```python
from build123d import *

# Parameters (mm, degrees)
SKETCH_2_R          = 1.05
EXTRUDE_1_DEPTH     = 6
EXTRUDE_3_DEPTH     = 10
SKETCH_5_R          = 1.75
CUT_EXTRUDE_1_DEPTH = 20.293781382
SKETCH_6_W          = 13
SKETCH_6_H          = 13
CUT_EXTRUDE_2_DEPTH = 1.5


with BuildPart() as part:
    # 草图2 → 凸台-拉伸1 (new body)
    with BuildSketch(Plane(origin=(0, 0, 0), x_dir=(1, 0, 0), z_dir=(0, 1, 0))):
        Polygon((-6.5, 3.25), (6.5, 3.25), (6.5, -6.75), (3.5, -9.75), (-6.5, -9.75), align=None)
        with Locations(Location((-3.25, 0, 0), (0, 0, 270))):
            Circle(SKETCH_2_R, mode=Mode.SUBTRACT)
        with Locations(Location((3.25, 0, 0), (0, 0, 270))):
            Circle(SKETCH_2_R, mode=Mode.SUBTRACT)
        with Locations(Location((-3.25, -6.5, 0), (0, 0, 270))):
            Circle(SKETCH_2_R, mode=Mode.SUBTRACT)
    extrude(amount=EXTRUDE_1_DEPTH)

    # 草图4 → 凸台-拉伸3 (add)
    with BuildSketch(Plane(origin=(6.5, 0, 11.5), x_dir=(0, 0, -1), z_dir=(1, 0, 0))):
        Polygon((9.75, 6), (9.75, 4.5), (10.95, 4.5), (10.95, 1.5), (9.75, 1.5), (9.75, 0), (6.75, 0), (6.75, 6), align=None)
    extrude(amount=EXTRUDE_3_DEPTH)

    # 草图5 → 切除-拉伸1 (cut, through all)
    with BuildSketch(Plane.XY.offset(4.75)):
        with Locations((10.5, 3)):
            Circle(SKETCH_5_R)
    extrude(amount=-CUT_EXTRUDE_1_DEPTH, mode=Mode.SUBTRACT)

    # 草图6 → 切除-拉伸2 (cut)
    with BuildSketch(Plane(origin=(0, 6, 0), x_dir=(1, 0, 0), z_dir=(0, 1, 0))):
        with Locations((0, -3.25)):
            Rectangle(SKETCH_6_W, SKETCH_6_H)
    extrude(amount=-CUT_EXTRUDE_2_DEPTH, mode=Mode.SUBTRACT)


solid = part.part
```
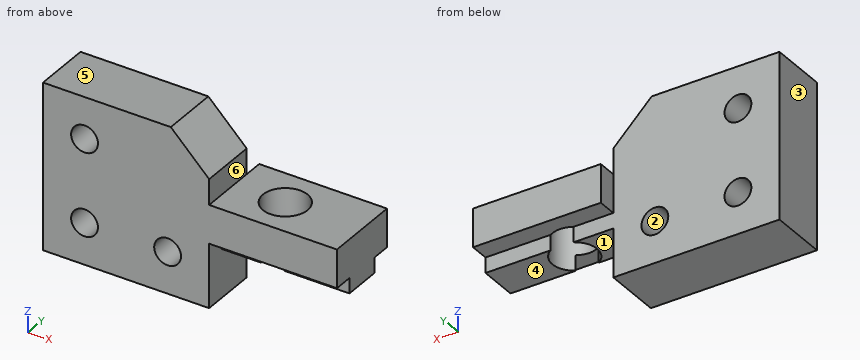
Geometry check sheet. Reference: the model listing, model coordinates, mm. Face numbers are marked on the shaded views. A direction names the side the tool comes from. Round coordinates to 2 decimals unless told otherwise and drop trailing zeros. Write each loop counter-clockwise with the first axis right and the second up, starting at its lowest first coordinate (ties: lowest second). Pieces come first, ordered by that corner, then holes. Notation, with made-up numbers: (6.25, -28) -> (32.25, -28) arc R18 ccw to (32.25, -7) -> close; hole circle Ø10 at (57, -18). An arc over 180 degrees is marked (long way). Put each result on its own line as item: value.
1) Cross-section at C-C, the plane z = 2.75. Enter the section's corners in (x, y).
Recorded:
outline: (-6.5, 0) -> (16.5, 0) -> (16.5, 6) -> (6.5, 6) -> (6.5, 4.5) -> (-6.5, 4.5) -> close; hole circle Ø3.5 at (10.5, 3)
2) Release check for a two-part mould opening along Z. For the marked faces 1, 2 and 3 record: pulls with the +Z half, pulls with the -Z half, needs draft (parallel to the pull), parting line crosses it, or undercut.
Recorded:
face 1: pulls with the -Z half
face 2: undercut
face 3: needs draft
3) Depth check by flat-ended pin: P1, Ø1, axis at y = 2.5, z = 6, coming from the +X side; P2, Ø4, axis at x = 3, z = 0, coming from the -Y side; P3, Ø1.3, axis at x = 14.5, z = 1, coming from the -Y side; P4, Ø2.5, axis at x = 14.5, y = 3, coming from the -Z side. Enter the tip coordinate at first touch or a pass-through.
Recorded:
P1: stops at x = 6.5
P2: stops at y = 0
P3: stops at y = 1.5
P4: stops at z = 0.55
4) Cross-section at A-A, the plane y = 3. Enter the section's corners in (x, z).
Recorded:
outline: (-6.5, -3.25) -> (6.5, -3.25) -> (6.5, 0.55) -> (8.75, 0.55) -> (8.75, 4.75) -> (6.5, 4.75) -> (6.5, 6.75) -> (3.5, 9.75) -> (-6.5, 9.75) -> close; (12.25, 0.55) -> (16.5, 0.55) -> (16.5, 4.75) -> (12.25, 4.75) -> close; hole circle Ø2.1 at (-3.25, 0); hole circle Ø2.1 at (-3.25, 6.5); hole circle Ø2.1 at (3.25, 0)
5) Cross-section at B-B, the plane x = 10.5. Enter the section's corners in (y, z).
Recorded:
outline: (0, 1.75) -> (1.25, 1.75) -> (1.25, 4.75) -> (0, 4.75) -> close; (4.75, 1.75) -> (6, 1.75) -> (6, 4.75) -> (4.75, 4.75) -> close
6) Cross-section at D-D, the plane y = 0.9. Enter the section's corners in (x, z).
Recorded:
outline: (-6.5, -3.25) -> (6.5, -3.25) -> (6.5, 1.75) -> (16.5, 1.75) -> (16.5, 4.75) -> (6.5, 4.75) -> (6.5, 6.75) -> (3.5, 9.75) -> (-6.5, 9.75) -> close; hole circle Ø2.1 at (-3.25, 0); hole circle Ø2.1 at (-3.25, 6.5); hole circle Ø2.1 at (3.25, 0)
7) Access from +Z, -Z, +X, -X, +Y, -Y to the whole of each face (thin tool, end or side, straight path). Record for the marked faces 4, 5 and 6.
Recorded:
face 4: -Z, +X, +Y, -Y
face 5: +Z, +X, -X, +Y, -Y
face 6: +Z, +X, +Y, -Y
8) Thickness scan on probe 1 along X at (y, z) = (1.1, 0); probe 2 along Z at (x, y) = (-3.25, 1.8); probe 3 along X at (y, z) = (2.25, -0.75). Record the ranges inside material, lowest first. Write a range as from..to.
Recorded:
probe 1: x = -6.5..-4.3, -2.2..2.2, 4.3..6.5
probe 2: z = -3.25..-1.05, 1.05..5.45, 7.55..9.75
probe 3: x = -6.5..-3.98, -2.52..2.52, 3.98..6.5
